Verification items for the finished model (mm, model axes). Round coordinates to 2 decimals unless told otherwise and drop trailing zeros. Order: outer loops, then holes, each group sorted by start corner. A loop starts at its lowest first (then second) coordinate and runs counter-clockwise, first axis right, second up.
```python
from build123d import *

# Parameters (mm, degrees)
BOSS_EXTRUDE1_DEPTH = 3
SKETCH2_R           = 0.9
CUT_EXTRUDE1_DEPTH  = 3


with BuildPart() as part:
    # Sketch1 → Boss-Extrude1 (new body)
    with BuildSketch(Plane.XY):
        Polygon((-17.596228945, -24.016474641), (17.403490925, -24.156507009), (28.352177859, 9.08693226), (0.119118647, 29.772539999), (-28.278558486, 9.313509391), align=None)
    extrude(amount=BOSS_EXTRUDE1_DEPTH)

    # Sketch2 → Cut-Extrude1 (cut)
    with BuildSketch(Plane(origin=(0, 0, 0), x_dir=(-1, 0, 0), z_dir=(0, 0, -1))):
        with Locations((2.651650429, -2.651650429)):
            Circle(SKETCH2_R)
        with Locations((-2.651650429, -2.651650429)):
            Circle(SKETCH2_R)
        with Locations((-2.651650429, 2.651650429)):
            Circle(SKETCH2_R)
        with Locations((2.651650429, 2.651650429)):
            Circle(SKETCH2_R)
    extrude(amount=-CUT_EXTRUDE1_DEPTH, mode=Mode.SUBTRACT)


solid = part.part
```
1) Scan lines: probe 1 along X at (y, z) = (-2.5, 1.05); probe 2 along X at (y, z) = (-15, 1.25); probe 3 along X at (y, z) = (19, 1.95). Record each from-to range of solid material in increasing order.
2) Draft check along X on faces 1 (the flat face through (14.433, 19.285, 1.479)), 2 (the cylindrical face through (-3.067, 1.853, 1.479)), 3 (the flat face through (-13.881, 19.686, 1.479)). Enter one of: released by +X, released by -X, zero draft, split by the parting line, or undercut.
3) Sectioned sample at B-B on z = 2.5. Record the cut outline in (x, y), then the cut area to 3 significant figures.
4) Sectioned sample at A-A on x = -2.5. Record the cut outline in (y, z).
5) Sectioned sample at C-C on y = 14.5. Record the cut outline in (x, z).
6) Go/stop test with a flat-tipped pin: pin 1 Ø2.5 at (x, y) = (-2.65, 2.65) entering from -Z. Record where the tip stops, or that it passes through.
7) Sectioned sample at D-D on x = 8. Record the cut outline in (y, z), then the cut area to 3 significant figures.
Returned:
1. probe 1: x = -24.49 to -3.54, -1.76 to 1.76, 3.54 to 24.54
1. probe 2: x = -20.49 to 20.42
1. probe 3: x = -14.83 to 14.82
2. face 1: released by +X
2. face 2: undercut
2. face 3: released by -X
3. outline: (-28.28, 9.31) - (-17.6, -24.02) - (17.4, -24.16) - (28.35, 9.09) - (0.12, 29.77) - close; hole circle Ø1.8 at (-2.65, -2.65); hole circle Ø1.8 at (-2.65, 2.65); hole circle Ø1.8 at (2.65, -2.65); hole circle Ø1.8 at (2.65, 2.65)
3. area: 2,100 mm2
4. outline: (-24.08, 0) - (-3.54, 0) - (-3.54, 3) - (-24.08, 3) - close; (-1.76, 0) - (1.76, 0) - (1.76, 3) - (-1.76, 3) - close; (3.54, 0) - (27.89, 0) - (27.89, 3) - (3.54, 3) - close
5. outline: (-21.08, 0) - (20.96, 0) - (20.96, 3) - (-21.08, 3) - close
6. pin 1: stops at z = 0
7. outline: (-24.12, 0) - (24, 0) - (24, 3) - (-24.12, 3) - close
7. area: 144 mm2
